Geometry: final body of the model. Coordinates: model frame, mm. Face numbers are marked on the shaded views. A direction names the side the tool comes from. Coordinates: 2 decimals unless noted, no trailing zeros. Loops run counter-clockwise (first coordinate to the right, second up) from the corner with the lowest first, then second, coordinate; pieces in that order, holes last. Notation, with made-up numbers: M 64.25,-12.5 L 123.25,-12.5 A27 cw 123.25,16.5 Z; hole C 30.25,26.25 d9. An arc over 180 degrees is marked long. Write item = value, one per line. Start each with the question number.
```python
from build123d import *

# Parameters (mm, degrees)
F0_W          = 5.842
F0_H          = 12.7
F0_R          = 3.175
F2_DEPTH      = 3.175
F3_R          = 1.7344184536
F4_DEPTH      = 6.35
F4_DEPTH_BACK = 1.27
F5_DEPTH      = 56.134
F6_R          = 2.6798601648
F7_DEPTH      = 25.4
F8_R          = 2.0084495131
F9_DEPTH      = 25.4


with BuildPart() as f1:
    # F0 (on Front) → F1 (revolve)
    with BuildSketch(Plane.XZ):
        Polygon((5.842, 12.7), (5.842, 0), (66.294, 0), (66.294, 12.7), (56.134, 12.7), (56.134, 10.16), (10.16, 10.16), (10.16, 12.7), align=None)
        with Locations((2.921, 6.35)):
            Rectangle(F0_W, F0_H)
    revolve(axis=Axis((33.147, 0, 0), (-1, 0, 0)))

    # F0 (on Front) → F2 (join, symmetric)
    with BuildSketch(Plane.XZ):
        with Locations((2.921, 6.35)):
            Rectangle(F0_W, F0_H)
        with BuildLine():
            Line((-0.9398, 0), (0, 0))
            Line((0, 0), (0, 12.7))
            Line((0, 12.7), (5.842, 12.7))
            Line((5.842, 12.7), (5.842, 15.24))
            Line((5.842, 15.24), (-0.508, 15.24))
            Line((-0.508, 15.24), (-10.8806298187, 3.8475430269))
            ThreePointArc((-10.8806298187, 3.8475430269), (-4.5919612295, 5.3297205562), (-0.9398, 0))
        make_face()
        with BuildLine():
            Line((5.842, 0), (0, 0))
            Line((0, 0), (-0.9398, 0))
            ThreePointArc((-0.9398, 0), (-3.1957909266, -4.5493385486), (-8.1826630726, -5.5069827884))
            Line((-8.1826630726, -5.5069827884), (5.842, -9.398))
            Line((5.842, -9.398), (5.842, 0))
        make_face()
        with BuildLine():
            ThreePointArc((-8.1826630726, -5.5069827884), (-3.1957909266, -4.5493385486), (-0.9398, 0))
            ThreePointArc((-0.9398, 0), (-4.5919612295, 5.3297205562), (-10.8806298187, 3.8475430269))
            ThreePointArc((-10.8806298187, 3.8475430269), (-12.1459778134, -1.5837270034), (-8.1826630726, -5.5069827884))
        make_face()
        with Locations((-6.6548, 0)):
            Circle(F0_R, mode=Mode.SUBTRACT)
    extrude(amount=F2_DEPTH, both=True)

    # F3 (on face) → F4 (join, two sides)
    with BuildSketch(Plane.YZ.offset(66.294)) as f4_sk:
        with BuildLine():
            ThreePointArc((-4.7824184536, 0), (0, -4.7824184536), (4.7824184536, 0))
            ThreePointArc((4.7824184536, 0), (0, 4.7824184536), (-4.7824184536, 0))
        make_face()
        Circle(F3_R, mode=Mode.SUBTRACT)
        with BuildLine():
            ThreePointArc((-4.7824184536, 0), (0, 4.7824184536), (4.7824184536, 0))
            Line((4.7824184536, 0), (4.7824184536, 15.24))
            Line((4.7824184536, 15.24), (-4.7824184536, 15.24))
            Line((-4.7824184536, 15.24), (-4.7824184536, 0))
        make_face()
    extrude(amount=F4_DEPTH)
    extrude(f4_sk.sketch, amount=-F4_DEPTH_BACK)

    # F5 (cut, through all): a face of the model
    f5_faces = [f1.faces().sort_by_distance(p)[0] for p in [
        (66.294, 0, 0),
    ]]
    extrude(f5_faces, amount=-F5_DEPTH, mode=Mode.SUBTRACT)

    # F6 (on face) → F7 (cut)
    with BuildSketch(Plane.XY.offset(15.24)):
        with Locations((68.6287283897, 0)):
            Circle(F6_R)
    extrude(amount=-F7_DEPTH, mode=Mode.SUBTRACT)

    # F8 (on face) → F9 (cut)
    with BuildSketch(Plane.XY.offset(15.24)):
        with Locations((2.5553756859, -0.2507429745)):
            Circle(F8_R)
    extrude(amount=-F9_DEPTH, mode=Mode.SUBTRACT)


solid = f1.part
```
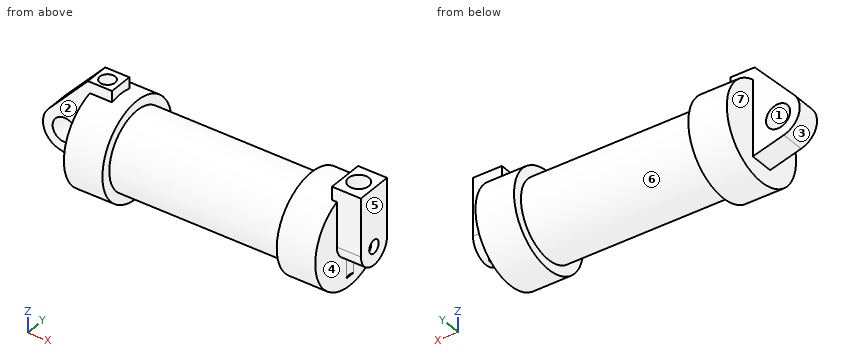
Item 1: Pull-direction query (X, two-part tool) for the marked faces 1, 2 and 3; classes: released by +X, released by -X, zero draft, split by the parting line, or undercut.
Item 2: Section query A-A (x = 42.5). Return the cut outline in (y, z), plus the area to 3 significant figures.
Item 3: Section query D-D (y = 6.25). Return the cut outline in (x, z).
Item 4: Reachability of the marked faces 4, 5, 6 and 7 from +Z, -Z, +X, -X, +Y, -Y: full face, straight path, thin tool, end or side. Return the list, or none.
Item 5: Section query B-B (z = 9.25). Return the cut outline in (x, y) (3 decimals), plus the area to 3 significant figures.
Item 6: Section query C-C (x = -7). Return the cut outline in (y, z) (3 decimals), plus the area to 3 significant figures.
Item 7: Line query: line 1 (X direction, y = -6.5, z = -8); line 2 (X direction, y = 0, z = 8.75); line 3 (X direction, y = 0, z = 8.25). Output: solid intervals per line, ascending. Write a range as from..to.
Item 8: First-contact query: pin 1 (12 mm diameter, centred on x = 11.5, z = -7.5, fed in from +Y); pin 2 (1 mm diameter, centred on y = -1, z = 13, fed in from -X); pin 3 (4 mm diameter, centred on x = 19, z = -5.5, fed in from -Y). Flat tips, straight axial feed; report the tip coordinate or a pass-through.
Verdict:
q1.face_1 = undercut
q1.face_2 = zero draft
q1.face_3 = released by -X
q2.outline = C 0,0 d20.32; hole C 0,0 d3.47
q2.area = 315 mm2
q3.outline = M 0,-11.06 L 10.16,-11.06 L 10.16,-8.01 L 56.13,-8.01 L 56.13,-11.06 L 66.29,-11.06 L 66.29,11.06 L 56.13,11.06 L 56.13,8.01 L 10.16,8.01 L 10.16,11.06 L 0,11.06 Z
q4.face_4 = -Z, +X
q4.face_5 = +Z, -Z, +X, +Y, -Y
q4.face_6 = none
q4.face_7 = -Z, -X
q5.outline = M -5.962,-3.175 L 0,-3.175 L 0,-8.702 L 10.16,-8.702 L 10.16,-4.203 L 56.134,-4.203 L 56.134,-8.702 L 66.294,-8.702 L 66.294,-4.782 L 72.644,-4.782 L 72.644,4.782 L 66.294,4.782 L 66.294,8.702 L 56.134,8.702 L 56.134,4.203 L 10.16,4.203 L 10.16,8.702 L 0,8.702 L 0,3.175 L -5.962,3.175 Z; hole C 2.555,-0.251 d4.017; hole C 68.629,0 d5.36
q5.area = 803 mm2
q6.outline = M -3.175,-5.835 L 3.175,-5.835 L 3.175,-3.156 L -3.175,-3.156 Z; M -3.175,3.156 L 3.175,3.156 L 3.175,8.11 L -3.175,8.11 Z
q6.area = 48.5 mm2
q7.line_1 = 0..10.16, 56.13..66.29
q7.line_2 = -6.42..0.56, 4.55..65.95, 71.31..72.64
q7.line_3 = -6.87..0.56, 4.55..65.95, 71.31..72.64
q8.pin_1 = 12.59
q8.pin_2 = -3
q8.pin_3 = -9.54
